Here's how the part is built. I have some questions about the finished solid (model axes, mm). A direction names the side the tool comes from. Round coordinates to 2 decimals unless told otherwise and drop trailing zeros. Order: outer loops, then holes, each group sorted by start corner. A loop starts at its lowest first (then second) coordinate and runs counter-clockwise, first axis right, second up.
```python
from build123d import *

# Parameters (mm, degrees)
SKETCH1_W               = 85.09
SKETCH1_H               = 40.64
SKETCH1_W_2             = 69.85
SKETCH1_H_2             = 25.4
BOSS_EXTRUDE1_DEPTH     = 12.7
SKETCH2_W               = 7.62
SKETCH2_H               = 7.62
SKETCH2_W_2             = 12.7
BOSS_EXTRUDE2_DEPTH     = 38.1
SKETCH4_W               = 85.09
SKETCH4_H               = 40.64
SKETCH4_W_2             = 69.85
SKETCH4_H_2             = 25.4
BOSS_EXTRUDE3_DEPTH     = 12.7
SKETCH6_W               = 12.7
SKETCH6_H               = 40.64
BOSS_EXTRUDE4_DEPTH     = 2.54
SKETCH7_W               = 12.7
SKETCH7_H               = 5.08
BOSS_EXTRUDE5_DEPTH     = 25.4
SKETCH8_W               = 6.35
SKETCH8_H               = 5.08
REVOLVE2_ANGLE          = 180
SKETCH10_R              = 2.0955
CUT_EXTRUDE4_DEPTH      = 32.4325
M4X0_7_TAPPED_HOLE1_D   = 3.3
SKETCH17_R              = 2.0955
BOSS_EXTRUDE6_DEPTH     = 9.2075
SKETCH18_R              = 2.0955
BOSS_EXTRUDE7_DEPTH     = 6.35
SKETCH24_W              = 63.5
SKETCH24_H              = 20.32
CUT_EXTRUDE9_DEPTH      = 32.75
CUT_EXTRUDE9_DEPTH_BACK = 86.09
CUT_EXTRUDE10_REACH     = 22.32
SKETCH25_R              = 2


with BuildPart() as part:
    # Sketch1 → Boss-Extrude1 (new body)
    with BuildSketch(Plane.XY):
        Rectangle(SKETCH1_W, SKETCH1_H)
        Rectangle(SKETCH1_W_2, SKETCH1_H_2, mode=Mode.SUBTRACT)
    extrude(amount=-BOSS_EXTRUDE1_DEPTH)

    # Sketch2 → Boss-Extrude2 (add)
    with BuildSketch(Plane(origin=(0, 0, -12.7), x_dir=(-1, 0, 0), z_dir=(0, 0, -1))):
        with Locations((-38.735, 16.51)):
            Rectangle(SKETCH2_W, SKETCH2_H)
        with Locations((-1.026508909, 16.51)):
            Rectangle(SKETCH2_W_2, SKETCH2_H)
        with Locations((38.735, 16.51)):
            Rectangle(SKETCH2_W, SKETCH2_H)
        with Locations((38.735, -16.51)):
            Rectangle(SKETCH2_W, SKETCH2_H)
        with Locations((-1.026508909, -16.51)):
            Rectangle(SKETCH2_W_2, SKETCH2_H)
        with Locations((-38.735, -16.51)):
            Rectangle(SKETCH2_W, SKETCH2_H)
    extrude(amount=BOSS_EXTRUDE2_DEPTH)

    # Sketch4 → Boss-Extrude3 (add)
    with BuildSketch(Plane(origin=(0, 0, -50.8), x_dir=(-1, 0, 0), z_dir=(0, 0, -1))):
        Rectangle(SKETCH4_W, SKETCH4_H)
        Rectangle(SKETCH4_W_2, SKETCH4_H_2, mode=Mode.SUBTRACT)
    extrude(amount=BOSS_EXTRUDE3_DEPTH)

    # Sketch6 → Boss-Extrude4 (add)
    with BuildSketch(Plane.ZY.offset(42.545)):
        with Locations((-31.75, 0)):
            Rectangle(SKETCH6_W, SKETCH6_H)
    extrude(amount=-BOSS_EXTRUDE4_DEPTH)

    # Sketch7 → Boss-Extrude5 (add)
    with BuildSketch(Plane.ZY.offset(42.545)):
        with Locations((-31.75, 8.5725)):
            Rectangle(SKETCH7_W, SKETCH7_H)
        with Locations((-31.75, -8.5725)):
            Rectangle(SKETCH7_W, SKETCH7_H)
    extrude(amount=BOSS_EXTRUDE5_DEPTH)

    # Sketch8 → Revolve2 (revolve)
    with BuildSketch(Plane.ZY.offset(67.945)):
        with Locations((-28.575, 8.5725)):
            Rectangle(SKETCH8_W, SKETCH8_H)
        with Locations((-28.575, -8.5725)):
            Rectangle(SKETCH8_W, SKETCH8_H)
    revolve(axis=Axis((-67.945, 11.1125, -31.75), (0, -1, 0)), revolution_arc=REVOLVE2_ANGLE)

    # Sketch10 → Cut-Extrude4 (cut, through all)
    with BuildSketch(Plane(origin=(0, 11.1125, 0), x_dir=(1, 0, 0), z_dir=(0, 1, 0))):
        with Locations((-67.945, 31.75)):
            Circle(SKETCH10_R)
    extrude(amount=-CUT_EXTRUDE4_DEPTH, mode=Mode.SUBTRACT)

    # M4x0.7 Tapped Hole1 (through all)
    with Locations(Plane(origin=(0, 20.32, 0), x_dir=(1, 0, 0), z_dir=(0, 1, 0))):
        with Locations((-14.101699785, 57.15), (15.108300215, 57.15), (15.108300215, 6.35), (-14.101699785, 6.35)):
            Hole(M4X0_7_TAPPED_HOLE1_D / 2)

    # Sketch17 → Boss-Extrude6 (add)
    with BuildSketch(Plane(origin=(0, 11.1125, 0), x_dir=(1, 0, 0), z_dir=(0, 1, 0))):
        with BuildLine():
            Line((-67.945, 25.4), (-42.545, 25.4))
            Line((-42.545, 25.4), (-42.545, 38.1))
            Line((-42.545, 38.1), (-67.945, 38.1))
            ThreePointArc((-67.945, 38.1), (-74.295, 31.75), (-67.945, 25.4))
        make_face()
        with Locations((-67.945, 31.75)):
            Circle(SKETCH17_R, mode=Mode.SUBTRACT)
    extrude(amount=BOSS_EXTRUDE6_DEPTH)

    # Sketch18 → Boss-Extrude7 (add)
    with BuildSketch(Plane.XZ.offset(11.1125)):
        with BuildLine():
            Line((-42.545, -38.1), (-42.545, -25.4))
            Line((-42.545, -25.4), (-67.945, -25.4))
            ThreePointArc((-67.945, -25.4), (-74.295, -31.75), (-67.945, -38.1))
            Line((-67.945, -38.1), (-42.545, -38.1))
        make_face()
        with Locations((-67.945, -31.75)):
            Circle(SKETCH18_R, mode=Mode.SUBTRACT)
    extrude(amount=BOSS_EXTRUDE7_DEPTH)

    # Sketch24 → Cut-Extrude9 (cut, two sides)
    with BuildSketch(Plane.ZY.offset(42.545)) as cut_extrude9_sk:
        with Locations((-31.75, -10.16)):
            Rectangle(SKETCH24_W, SKETCH24_H)
    extrude(amount=CUT_EXTRUDE9_DEPTH, mode=Mode.SUBTRACT)
    extrude(cut_extrude9_sk.sketch, amount=-CUT_EXTRUDE9_DEPTH_BACK, mode=Mode.SUBTRACT)

    # Sketch25 → Cut-Extrude10 (cut, up to next)
    with BuildSketch(Plane(origin=(0, 20.32, 0), x_dir=(1, 0, 0), z_dir=(0, 1, 0)), mode=Mode.PRIVATE) as cut_extrude10_sk1:
        with Locations((38.735, 57.15)):
            Circle(SKETCH25_R)
    cut_extrude10_tool1 = extrude(cut_extrude10_sk1.sketch, amount=-CUT_EXTRUDE10_REACH, mode=Mode.PRIVATE) & part.part
    add(cut_extrude10_tool1.solids().sort_by_distance((38.735, 20.32, -57.15))[0], mode=Mode.SUBTRACT)
    # Sketch25 → Cut-Extrude10 (cut, up to next)
    with BuildSketch(Plane(origin=(0, 20.32, 0), x_dir=(1, 0, 0), z_dir=(0, 1, 0)), mode=Mode.PRIVATE) as cut_extrude10_sk2:
        with Locations((38.735, 6.35)):
            Circle(SKETCH25_R)
    cut_extrude10_tool2 = extrude(cut_extrude10_sk2.sketch, amount=-CUT_EXTRUDE10_REACH, mode=Mode.PRIVATE) & part.part
    add(cut_extrude10_tool2.solids().sort_by_distance((38.735, 20.32, -6.35))[0], mode=Mode.SUBTRACT)


solid = part.part
```
1) If we section it at B-B (y = 3.5): Write out the boundary of the cut face in (x, z) (3 decimals).
2) If we section it at C-C (x = -20): Write out the boundary of the cut face in (y, z).
3) If we section it at D-D (z = -31.75): Write out the boundary of the cut face in (x, y) (1 decimal).
4) For faces 1 (the flat face through (-42.545, 12, -53)), 2 (the flat face through (39, 6, -50.8)), 3 (the flat face through (-20, 17, -12.7)), which set-ups out of +Z, -Z, +X, -X, +Y, -Y let a thin tool reach every point of the face, with its end or its side?
5) I'm going to push flat-ended pins straight in: pin 1 (8.5 mm diameter, centred on y = 16.5, z = -35, fed in from -X) (3 decimals); pin 2 (6.5 mm diameter, centred on y = 2.5, z = -30.5, fed in from -X) (3 decimals); pin 3 (10 mm diameter, centred on y = 9, z = -26, fed in from -X); pin 4 (2 mm diameter, centred on y = 8.5, z = -48, fed in from -X). Where does each tip first touch, or does it pass through?
6) We'd pull the mould along X, two halves only. Please class faces 4 (the flat face through (34.925, 16, -31)), 5 (the flat face through (-34.925, 6, -57)), 6 (the flat face through (-42.545, 12, -10)), 7 (the flat face through (-59, 6.032, -32)): +X half, -X half, draft (parallel to the pull), parting line (faces both ways), or undercut.
7) I need wall thicknesses on line 1 (X direction, y = 14.25, z = -31.75) (1 decimal); line 2 (X direction, y = 5.75, z = -57) (3 decimals); line 3 (X direction, y = 14.5, z = -46.5) (1 decimal). Which ranges of each line are inside material? Lowest first, please.
8) If we section it at A-A (z = -23): Write out the boundary of the cut face in (x, y) (1 decimal), plus the area to 3 significant figures.
Solutions:
1. outline: (-42.545, -63.5) - (-34.925, -63.5) - (-34.925, -50.8) - (-42.545, -50.8) - close; (-42.545, -38.1) - (-40.005, -38.1) - (-40.005, -25.4) - (-42.545, -25.4) - close; (-42.545, -12.7) - (-34.925, -12.7) - (-34.925, 0) - (-42.545, 0) - close; (34.925, -63.5) - (42.545, -63.5) - (42.545, -50.8) - (34.925, -50.8) - close; (34.925, -12.7) - (42.545, -12.7) - (42.545, 0) - (34.925, 0) - close; hole circle Ø4 at (38.735, -57.15); hole circle Ø4 at (38.735, -6.35)
2. outline: (12.7, -63.5) - (20.32, -63.5) - (20.32, -50.8) - (12.7, -50.8) - close; (12.7, -12.7) - (20.32, -12.7) - (20.32, 0) - (12.7, 0) - close
3. outline: (-74.3, 6) - (-70, 6) - (-70, 20.3) - (-74.3, 20.3) - close; (-65.8, 6) - (-42.5, 6) - (-42.5, 0) - (-40, 0) - (-40, 12.7) - (-34.9, 12.7) - (-34.9, 20.3) - (-65.8, 20.3) - close; (-5.3, 12.7) - (7.4, 12.7) - (7.4, 20.3) - (-5.3, 20.3) - close; (34.9, 12.7) - (42.5, 12.7) - (42.5, 20.3) - (34.9, 20.3) - close
4. face 1: -Z, -X, +Y, -Y
4. face 2: +X, -X, -Y
4. face 3: +Y, -Y
5. pin 1: stops at x = -74.295
5. pin 2: stops at x = -42.545
5. pin 3: stops at x = -74.25
5. pin 4: passes through
6. face 4: undercut
6. face 5: undercut
6. face 6: -X half
6. face 7: draft
7. line 1: x = -74.3 to -70, -65.8 to -34.9, -5.3 to 7.4, 34.9 to 42.5
7. line 2: x = -42.545 to -34.925, 34.925 to 36.741, 40.729 to 42.545
7. line 3: x = -42.5 to -34.9, -5.3 to 7.4, 34.9 to 42.5
8. outline: (-42.5, 12.7) - (-34.9, 12.7) - (-34.9, 20.3) - (-42.5, 20.3) - close; (-5.3, 12.7) - (7.4, 12.7) - (7.4, 20.3) - (-5.3, 20.3) - close; (34.9, 12.7) - (42.5, 12.7) - (42.5, 20.3) - (34.9, 20.3) - close
8. area: 213 mm2
